CAD build for the part. Positions are in the model's coordinates, mm. A direction names the side the tool comes from. Give positions to 0.01 mm unless a question says otherwise; leave off trailing zeros. Order: outer loops, then holes, each group sorted by start corner. A loop starts at its lowest first (then second) coordinate and runs counter-clockwise, first axis right, second up. Notation, with made-up numbers: M -32.5,-39.5 L 13.5,-39.5 A16 ccw 13.5,-27.5 Z; hole C 21,37 d10. An arc over 180 degrees is marked long. Put each result on its own line as item: value. Start each with the question number.
1) Cut at C-C (x = 42.5). Write the cut outline in (y, z).
2) Cut at A-A (z = -117). Write the cut outline in (x, y), and give its area (3 significant figures).
3) Cut at B-B (y = -2.5). Write the cut outline in (x, z).
4) Pin check, flat tip, straight feed: pin 1 (3 mm diameter, centred on x = -75, z = 27.5, fed in from +Y). Stop position of the tip, or through.
5) Two-plate mould, pull along X, no slides. Class faces 1 (the face through (76.2, -3, -104)), 2 (the face through (-101.6, -3, -11)), 3 (the face through (66, 0, -11)), 4 (the face through (63.5, -3, -12)): released by +X, released by -X, zero draft, split by the parting line, or undercut.
6) Drill centre lines: line 1 (Z direction, x = -31, y = -0.75); line 2 (X direction, y = -0.75, z = -124); line 3 (Z direction, x = 6.5, y = -5.25). Where is each one in solid material? Low to high. Write a range as [from, to].
7) Tool access for faces 5 (the face through (66, -6.35, -11)), 6 (the face through (70, -3, 53.243)): list every direction of +Z, -Z, +X, -X, +Y, -Y with a clear straight run to the whole face (end or side of a thin tool).
```python
from build123d import *

# Parameters (mm, degrees)
F1_DEPTH = 6.35


with BuildPart() as f1:
    # F0 (on Front) → F1 (new body)
    with BuildSketch(Plane.XZ):
        Polygon((76.2, -129.44348), (101.6, -129.44348), (101.6, 129.44348), (-101.6, 129.44348), (-101.6, -129.44348), (-76.2, -129.44348), (-76.2, -78.64348), (-63.5, -78.64348), (-63.5, 53.24348), (-76.2, 53.24348), (-76.2, 104.04348), (-25.4, 104.04348), (-25.4, 91.34348), (25.4, 91.34348), (25.4, 104.04348), (76.2, 104.04348), (76.2, 53.24348), (63.5, 53.24348), (63.5, -78.64348), (76.2, -78.64348), align=None)
        Polygon((101.6, -154.84348), (101.6, -129.44348), (76.2, -129.44348), (63.5, -129.44348), (-63.5, -129.44348), (-76.2, -129.44348), (-101.6, -129.44348), (-101.6, -154.84348), align=None)
    extrude(amount=F1_DEPTH)


solid = f1.part
```
Solution:
1. outline: M -6.35,-154.84 L 0,-154.84 L 0,-129.44 L -6.35,-129.44 Z; M -6.35,104.04 L 0,104.04 L 0,129.44 L -6.35,129.44 Z
2. outline: M -101.6,-6.35 L -76.2,-6.35 L -76.2,0 L -101.6,0 Z; M 76.2,-6.35 L 101.6,-6.35 L 101.6,0 L 76.2,0 Z
2. area: 323 mm²
3. outline: M -101.6,-154.84 L 101.6,-154.84 L 101.6,129.44 L -101.6,129.44 Z; hole M -76.2,-129.44 L 76.2,-129.44 L 76.2,-78.64 L 63.5,-78.64 L 63.5,53.24 L 76.2,53.24 L 76.2,104.04 L 25.4,104.04 L 25.4,91.34 L -25.4,91.34 L -25.4,104.04 L -76.2,104.04 L -76.2,53.24 L -63.5,53.24 L -63.5,-78.64 L -76.2,-78.64 Z
4. pin 1: y = 0
5. face 1: undercut
5. face 2: released by -X
5. face 3: zero draft
5. face 4: undercut
6. line 1: [-154.84, -129.44], [104.04, 129.44]
6. line 2: [-101.6, -76.2], [76.2, 101.6]
6. line 3: [-154.84, -129.44], [91.34, 129.44]
7. face 5: +Z, -Z, +X, -X, -Y
7. face 6: +Y, -Y
